Source: three-view drawing plus pictorial views. Frame: mm from the lowest corner of the part. Round coordinates to 2 decimals unless told otherwise and drop trailing zeros. Loops run counter-clockwise (first coordinate to the right, second up) from the corner with the lowest first, then second, coordinate; pieces in that order, holes last. Notation, with made-up numbers: M 24.5,52.25 L 35.5,52.25 A9 cw 35.5,65.25 Z; hole C 27,-36.5 d10. An arc over 180 degrees is marked long. Answer as a JSON object with one key per item and string values.
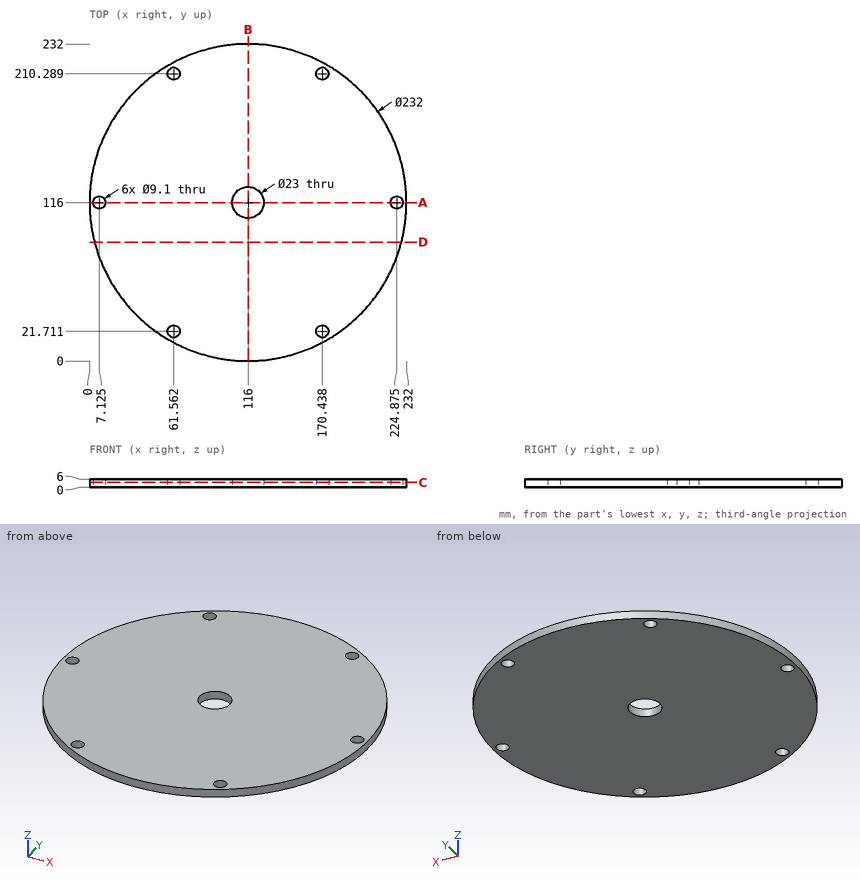
1) First-contact query: pin 1 (14 mm diameter, centred on x = 116, y = 116, fed in from +Z). Flat tip, straight axial feed; report the tip coordinate or a pass-through.
Geometry results:
{"pin 1": "through"}
2) Cut plane C-C on z = 3.45. Count the separate pieces of the cut face and the enclosed holes in it, and give its area (3 significant figures).
Geometry results:
{"separate pieces": "1", "enclosed holes": "7", "area": "41,500 mm2"}
3) Cut plane B-B on x = 116. Return the cut outline in (y, z).
Geometry results:
{"outline": "M 0,0 L 104.5,0 L 104.5,6 L 0,6 Z; M 127.5,0 L 232,0 L 232,6 L 127.5,6 Z"}
4) Line query: probe 1 along Y at (x, z) = (116, 1.8); probe 2 along Y at (x, z) = (189.5, 4.15) (1 decimal); probe 3 along X at (y, z) = (118, 5) (1 decimal). Output: solid intervals per line, ascending.
Geometry results:
{"probe 1": "0 to 104.5, 127.5 to 232", "probe 2": "26.3 to 205.7", "probe 3": "0 to 3, 11.2 to 104.7, 127.3 to 220.8, 229 to 232"}
5) Cut plane A-A on y = 116. Return the cut outline in (x, z) (1 decimal).
Geometry results:
{"outline": "M 0,0 L 2.6,0 L 2.6,6 L 0,6 Z; M 11.7,0 L 104.5,0 L 104.5,6 L 11.7,6 Z; M 127.5,0 L 220.3,0 L 220.3,6 L 127.5,6 Z; M 229.4,0 L 232,0 L 232,6 L 229.4,6 Z"}
6) Cut plane D-D on y = 87. Return the cut outline in (x, z).
Geometry results:
{"outline": "M 3.68,0 L 228.32,0 L 228.32,6 L 3.68,6 Z"}
